```python
from build123d import *

# Parameters (mm, degrees)
SKETCH_1_W          = 25
SKETCH_1_H          = 20
EXTRUDE_1_DEPTH     = 1
EXTRUDE_2_DEPTH     = 1
EXTRUDE_3_DEPTH     = 1
SKETCH_5_W          = 19.8
SKETCH_5_H          = 14.8
EXTRUDE_4_DEPTH     = 1
SKETCH_6_R          = 2
CUT_EXTRUDE_2_DEPTH = 1.6
SKETCH_7_R          = 3
CUT_EXTRUDE_3_DEPTH = 1


with BuildPart() as part:
    # Эскиз1 → Бобышка-Вытянуть1 (new body)
    with BuildSketch(Plane(origin=(0, 0, 0), x_dir=(1, 0, 0), z_dir=(0, 1, 0))):
        Rectangle(SKETCH_1_W, SKETCH_1_H)
    extrude(amount=EXTRUDE_1_DEPTH)

    # Эскиз3 → Бобышка-Вытянуть2 (add)
    with BuildSketch(Plane(origin=(0, 0, 0), x_dir=(1, 0, 0), z_dir=(0, 1, 0))):
        Polygon((-14.5, 7.5), (-17.5, 7.5), (-17.5, -7.5), (-14.5, -7.5), (-12.5, -7.5), (-12.5, -6.5), (-14.5, -6.5), (-14.5, 6.5), (-12.5, 6.5), (-12.5, 7.5), align=None)
    extrude(amount=EXTRUDE_2_DEPTH)

    # Эскиз4 → Бобышка-Вытянуть3 (add)
    with BuildSketch(Plane(origin=(0, 0, 0), x_dir=(1, 0, 0), z_dir=(0, 1, 0))):
        with BuildLine():
            Line((9.5, 10), (9.5, 18))
            ThreePointArc((9.5, 18), (8.35, 19.15), (7.2, 18))
            Line((7.2, 18), (7.2, 17))
            ThreePointArc((7.2, 17), (6.614213562, 15.585786438), (5.2, 15))
            Line((5.2, 15), (-1.3, 15))
            Line((-1.3, 15), (-1.3, 14))
            Line((-1.3, 14), (-4.3, 14))
            Line((-4.3, 14), (-4.3, 17))
            Line((-4.3, 17), (-1.3, 17))
            Line((-1.3, 17), (-1.3, 16))
            Line((-1.3, 16), (5.2, 16))
            ThreePointArc((5.2, 16), (5.907106781, 16.292893219), (6.2, 17))
            Line((6.2, 17), (6.2, 18))
            ThreePointArc((6.2, 18), (8.35, 20.15), (10.5, 18))
            Line((10.5, 18), (10.5, 10))
            Line((10.5, 10), (9.5, 10))
        make_face()
        with BuildLine():
            Line((-4.3, -14), (-4.3, -17))
            Line((-4.3, -17), (-1.3, -17))
            Line((-1.3, -17), (-1.3, -16))
            Line((-1.3, -16), (5.2, -16))
            ThreePointArc((5.2, -16), (5.907106781, -16.292893219), (6.2, -17))
            Line((6.2, -17), (6.2, -18))
            ThreePointArc((6.2, -18), (8.35, -20.15), (10.5, -18))
            Line((10.5, -18), (10.5, -10))
            Line((10.5, -10), (9.5, -10))
            Line((9.5, -10), (9.5, -18))
            ThreePointArc((9.5, -18), (8.35, -19.15), (7.2, -18))
            Line((7.2, -18), (7.2, -17))
            ThreePointArc((7.2, -17), (6.614213562, -15.585786438), (5.2, -15))
            Line((5.2, -15), (-1.3, -15))
            Line((-1.3, -15), (-1.3, -14))
            Line((-1.3, -14), (-4.3, -14))
        make_face()
    extrude(amount=EXTRUDE_3_DEPTH)

    # Эскиз5 → Бобышка-Вытянуть4 (add)
    with BuildSketch(Plane(origin=(0, 1, 0), x_dir=(1, 0, 0), z_dir=(0, 1, 0))):
        Rectangle(SKETCH_5_W, SKETCH_5_H)
    extrude(amount=EXTRUDE_4_DEPTH)

    # Эскиз6 → Вырез-Вытянуть2 (cut)
    with BuildSketch(Plane.XZ):
        with Locations(Location((0, 0, 0), (0, 0, 270))):
            Circle(SKETCH_6_R)
    extrude(amount=-CUT_EXTRUDE_2_DEPTH, mode=Mode.SUBTRACT)

    # Эскиз7 → Вырез-Вытянуть3 (cut)
    with BuildSketch(Plane.XZ):
        with Locations((-6.25, -11.55)):
            Circle(SKETCH_7_R)
    extrude(amount=-CUT_EXTRUDE_3_DEPTH, mode=Mode.SUBTRACT)


solid = part.part
```
Can you work these out from the model? Positions are in its coordinate system, mm. A direction names the side the tool comes from. Coordinates: 2 decimals unless noted, no trailing zeros. Order: outer loops, then holes, each group sorted by start corner. A loop starts at its lowest first (then second) coordinate and runs counter-clockwise, first axis right, second up. Notation, with made-up numbers: (-13, 53.25) - (3, 53.25) arc R17 ccw to (3, 72.25) - close; hole circle Ø6 at (80, 8.5). An arc over 180 degrees is marked (long way). Answer in a Markdown table with one row per item.
1. For pin 1 (0.8 mm diameter, centred on x = -15.5, y = 0.5, fed in from +Z); pin 2 (1.1 mm diameter, centred on x = 11.5, y = 0.5, fed in from -Z); pin 3 (0.5 mm diameter, centred on x = -2.5, y = 0.5, fed in from -Z), each with a flat end and sliding along its axis, tell me the tip position at first contact or that it passes through.
Reply:
| item | result |
|---|---|
| pin 1 | stops at z = 7.5 |
| pin 2 | stops at z = -10 |
| pin 3 | stops at z = -17 |
2. Suppose I cut it at C-C (x = 8.35). Please give me the cut outline in (y, z), and give its area (3 significant figures).
Reply:
| item | result |
|---|---|
| outline | (0, -20.15) - (1, -20.15) - (1, -19.15) - (0, -19.15) - close; (0, -10) - (1, -10) - (1, -7.4) - (2, -7.4) - (2, 7.4) - (1, 7.4) - (1, 10) - (0, 10) - close; (0, 19.15) - (1, 19.15) - (1, 20.15) - (0, 20.15) - close |
| area | 36.8 mm^2 |
3. Suppose I cut it at A-A (x = 0). Please give me the cut outline in (y, z).
Reply:
| item | result |
|---|---|
| outline | (0, -16) - (1, -16) - (1, -15) - (0, -15) - close; (0, -10) - (1, -10) - (1, -7.4) - (2, -7.4) - (2, 7.4) - (1, 7.4) - (1, 10) - (0, 10) - (0, 2) - (1.6, 2) - (1.6, -2) - (0, -2) - close; (0, 15) - (1, 15) - (1, 16) - (0, 16) - close |
4. If I drill on line 1 along X through (y, z) = (0.8, 0); line 2 along Z through (x, y) = (3.75, 0.5); line 3 along X through (y, z) = (1.05, 0), over which ranges is the centre line in solid material (lowest first)?
Reply:
| item | result |
|---|---|
| line 1 | x = -17.5 to -14.5, -12.5 to -2, 2 to 12.5 |
| line 2 | z = -16 to -15, -10 to 10, 15 to 16 |
| line 3 | x = -9.9 to -2, 2 to 9.9 |
5. For faces 4 (the flat face through (-12.5, 0.5, -8.7)), 5 (the flat face through (-1.7, 0.5, 10)), 6 (the flat face through (9.5, 0.5, -13.9)), which set-ups out of +Z, -Z, +X, -X, +Y, -Y let a thin tool reach every point of the face, with its end or its side?
Reply:
| item | result |
|---|---|
| face 4 | -Z, -X, +Y, -Y |
| face 5 | -X, +Y, -Y |
| face 6 | +Y, -Y |
6. Suppose I cut it at D-D (y = 0.5). Give the number of separate pieces and of enclosed holes in the cut face, and give its area (3 significant figures).
Reply:
| item | result |
|---|---|
| separate pieces | 1 |
| enclosed holes | 2 |
| area | 595 mm^2 |
7. If we mould it in two halves opening along Z, with no side actions, what happens to faces 1 (the flat face through (-1.3, 0.5, -14.5)), 2 (the flat face through (10.5, 0.5, 14.1)), 3 (the flat face through (-2.8, 0.5, -17))? For each: pulls with the +Z half, pulls with the -Z half, needs draft (parallel to the pull), parting line crosses it, or undercut.
Reply:
| item | result |
|---|---|
| face 1 | undercut |
| face 2 | needs draft |
| face 3 | pulls with the -Z half |
8. Suppose I cut it at B-B (z = 0). Please give me the cut outline in (x, y).
Reply:
| item | result |
|---|---|
| outline | (-17.5, 0) - (-14.5, 0) - (-14.5, 1) - (-17.5, 1) - close; (-12.5, 0) - (-2, 0) - (-2, 1.6) - (2, 1.6) - (2, 0) - (12.5, 0) - (12.5, 1) - (9.9, 1) - (9.9, 2) - (-9.9, 2) - (-9.9, 1) - (-12.5, 1) - close |
